Input: part model. Units: mm. Frame: model coordinates. A direction names the side the tool comes from. Round coordinates to 2 decimals unless told otherwise and drop trailing zeros. Write each loop counter-clockwise with the first axis right and the second up, starting at its lowest first coordinate (ties: lowest second). Pieces come first, ordered by that corner, then holes. Notation, with made-up numbers: M -25,12 L 34,12 A28 ccw 34,39 Z; hole C -2.75,6 d3. An arc over 180 degrees is marked long. Answer as CSV lines item,"result". Start each with the question number.
```python
from build123d import *

# Parameters (mm, degrees)
SKETCH1_W           = 20.735936364
SKETCH1_H           = 3.175
BOSS_EXTRUDE1_DEPTH = 6.35
SKETCH2_W           = 82.651107169
SKETCH2_H           = 6.52720724
SKETCH2_W_2         = 76.969823319
SKETCH2_H_2         = 6.604
CUT_EXTRUDE1_DEPTH  = 7.35
SKETCH6_W           = 206.502
SKETCH6_H           = 3.711703494
SKETCH6_H_2         = 2.816288331
BOSS_EXTRUDE3_DEPTH = 31.75
BOSS_EXTRUDE5_DEPTH = 130.429


with BuildPart() as part:
    # Sketch1 → Boss-Extrude1 (new body)
    with BuildSketch(Plane(origin=(0, 0, 0), x_dir=(0, 0, -1), z_dir=(1, 0, 0))):
        Polygon((-123.525645009, 81.218983384), (-123.525645009, -25.082949612), (-102.22101814, -26.860004783), (-104.557017494, 0), (-79.646789796, 17.686261666), (-41.094549164, 17.686261666), (-13.779824281, -3.641289166), (-17.947471695, -33.889404663), (-12.561862574, -34.338627482), (90.228248196, -18.303088648), (90.228248196, 91.281577209), (0, 117.577378193), (-20.735936364, 117.577378193), align=None)
        Polygon((5.201841666, 40.001048477), (77.528248196, 55.056292197), (77.528248196, 85.830387495), (5.201841666, 105.015188817), align=None, mode=Mode.SUBTRACT)
        Polygon((-79.646789796, 84.224142025), (-79.646789796, 48.574048336), (0, 40.007327233), (0, 105.015188817), (-20.735936364, 105.015188817), align=None, mode=Mode.SUBTRACT)
        Polygon((-86.090479579, 81.218983384), (-86.090479579, 50.197772081), (-114.759972161, 55.666680192), (-114.759972161, 71.350976637), align=None, mode=Mode.SUBTRACT)
        with Locations((-10.367968182, 112.814878193)):
            Rectangle(SKETCH1_W, SKETCH1_H, mode=Mode.SUBTRACT)
    extrude(amount=BOSS_EXTRUDE1_DEPTH)

    # Sketch2 → Cut-Extrude1 (cut, through all)
    with BuildSketch(Plane(origin=(6.35, 0, 0), x_dir=(0, 0, -1), z_dir=(1, 0, 0))):
        with Locations((117.850801407, 29.125465717)):
            Rectangle(SKETCH2_W, SKETCH2_H)
        with Locations((-85.04073335, 29.163862097)):
            Rectangle(SKETCH2_W_2, SKETCH2_H_2)
    extrude(amount=-CUT_EXTRUDE1_DEPTH, mode=Mode.SUBTRACT)

    # Sketch6 → Boss-Extrude3 (add)
    with BuildSketch(Plane.ZY):
        with Locations((20.274645009, 34.244921084)):
            Rectangle(SKETCH6_W, SKETCH6_H)
        with Locations((20.274645009, 24.453717932)):
            Rectangle(SKETCH6_W, SKETCH6_H_2)
    extrude(amount=-BOSS_EXTRUDE3_DEPTH)

    # Sketch8 → Boss-Extrude5 (add)
    with BuildSketch(Plane.ZY):
        Polygon((0, 117.577378193), (-83.878248196, 93.218298083), (-90.228248196, 91.281577209), (-90.228248196, 32.389069337), (-83.878248196, 32.389069337), (-83.878248196, 86.868298083), (-9.525197863, 108.461165703), (29.097772116, 108.270149457), (123.542635704, 74.868983384), (123.525645009, 81.218983384), (20.735936364, 117.577378193), (20.752927059, 113.344232588), (26.228286967, 113.344232588), (26.228286967, 111.139694939), (20.752927059, 111.139694939), (0.016990695, 111.139694939), (-7.377605414, 111.139694939), (-7.377605414, 113.344232588), (0.011172356, 113.344232588), align=None)
    extrude(amount=-BOSS_EXTRUDE5_DEPTH)


solid = part.part
```
Item 1: Cut plane B-B, the plane z = -46. Return loops of the section in (x, y), plus the area to 3 significant figures.
Item 2: Cut plane C-C, the plane z = 49. Return loops of the section in (x, y), plus the area to 3 significant figures.
Item 3: Cut plane A-A, the plane y = 59.5. Return loops of the section in (x, z), plus the area to 3 significant figures.
Item 4: Draft query along Z for faces 4 (the face through (64.301, 92.263, -87.009)), 5 (the face through (3, 114.402, 11)), 6 (the face through (3.13, -25.96, 113.02)). Return one class per face: +Z half, -Z half, draft (parallel to the pull), parting line (faces both ways), or undercut.
Item 5: Line query: line 1 (Y direction, x = 9, z = 5); line 2 (Y direction, x = 15.5, z = 61); line 3 (Z direction, x = 17.5, y = 66). Output: solid intervals per line, ascending. Write a range as [from, to].
Item 6: Access query for faces 1 (the face through (64.301, 91.803, 75.659)), 2 (the face through (64, 61, -90.228)), 3 (the face through (3, 66, 86.09)). Directions: +Z, -Z, +X, -X, +Y, -Y. A direction counts if a zero-diameter tool reaches every point of the face in a straight line with its end or side. Return the directions, or none.
Item 7: Cut plane D-D, the plane x = 113. Return loops of the section in (y, z), plus the area to 3 significant figures.
Item 8: Pin query (flat end, axial travel): pin 1 Ø7 at (y, z) = (115, 3) entering from +X; pin 2 Ø6 at (x, z) = (40, -3.5) entering from -Y; pin 3 Ø3 at (x, z) = (80.5, -53) entering from -Y; pin 4 Ø1.5 at (x, y) = (53.5, 52) entering from +Z. Return the tip coordinate at first contact, or that it passes through.
Results list:
1,outline,"M 0,-25.2 L 6.35,-25.2 L 6.35,23.05 L 31.75,23.05 L 31.75,25.86 L 6.35,25.86 L 6.35,32.39 L 31.75,32.39 L 31.75,36.1 L 6.35,36.1 L 6.35,48.49 L 0,48.49 Z; M 0,94.19 L 6.35,94.19 L 6.35,97.87 L 130.43,97.87 L 130.43,104.22 L 0,104.22 Z"
1,area,"1,490 mm²"
2,outline,"M 0,17.69 L 6.35,17.69 L 6.35,23.05 L 31.75,23.05 L 31.75,25.86 L 0,25.86 Z; M 0,32.39 L 31.75,32.39 L 31.75,36.1 L 6.35,36.1 L 6.35,45.28 L 0,45.28 Z; M 0,95.04 L 6.35,95.04 L 6.35,101.23 L 130.43,101.23 L 130.43,107.58 L 0,107.58 Z"
2,area,"1,170 mm²"
3,outline,"M 0,-90.23 L 130.43,-90.23 L 130.43,-83.88 L 6.35,-83.88 L 6.35,-77.53 L 0,-77.53 Z; M 0,-5.2 L 6.35,-5.2 L 6.35,0 L 0,0 Z; M 0,79.65 L 6.35,79.65 L 6.35,86.09 L 0,86.09 Z; M 0,114.76 L 6.35,114.76 L 6.35,123.53 L 0,123.53 Z"
3,area,"998 mm²"
4,face 4,"-Z half"
4,face 5,"undercut"
4,face 6,"+Z half"
5,line 1,"[23.05, 25.86], [32.39, 36.1], [108.39, 111.14]"
5,line 2,"[23.05, 25.86], [32.39, 36.1], [96.99, 103.34]"
5,line 3,"[-90.23, -83.88]"
6,face 1,"+X"
6,face 2,"-Z, +X, -X, +Y, -Y"
6,face 3,"+X, -X"
7,outline,"M 32.39,-90.23 L 91.28,-90.23 L 93.22,-83.88 L 117.58,0 L 113.34,0.01 L 113.34,-7.38 L 111.14,-7.38 L 111.14,26.23 L 113.34,26.23 L 113.34,20.75 L 117.58,20.74 L 81.22,123.53 L 74.87,123.54 L 108.27,29.1 L 108.46,-9.53 L 86.87,-83.88 L 32.39,-83.88 Z"
7,area,"1,620 mm²"
8,pin 1,"x = 130.43"
8,pin 2,"y = 108.42"
8,pin 3,"y = 95.4"
8,pin 4,"z = -83.88"
